from build123d import *

# Parameters (mm, degrees)
F0_W     = 27
F0_H     = 12.6
F1_DEPTH = 4
F3_DEPTH = 25
F4_R     = 2
F6_DEPTH = 2
F7_SIZE2 = 2
F7_SIZE  = 1.8


with BuildPart() as f1:
    # F0 (on Top) → F1 (new body)
    with BuildSketch(Plane.XY):
        with Locations((13.5, 6.3)):
            Rectangle(F0_W, F0_H)
    extrude(amount=F1_DEPTH)

    # F2 (on face) → F3 (cut)
    with BuildSketch(Plane.XY.offset(4)):
        Polygon((11.3033894163, 10), (0, 10), (0, 2.6), (11.3033894163, 2.6), (15, 6.1416643043), align=None)
    extrude(amount=-F3_DEPTH, mode=Mode.SUBTRACT)

    # F4
    f4_edges = [f1.edges().sort_by_distance(p)[0] for p in [
        (11.303389, 10, 2),
        (15, 6.141664, 2),
        (11.303389, 2.6, 2),
    ]]
    fillet(f4_edges, radius=F4_R)

    # F5 (on face) → F6 (cut)
    with BuildSketch(Plane.XY.offset(4)):
        with BuildLine():
            Line((27, 12.6), (13, 12.6))
            Line((13, 12.6), (19.9540073999, 7.1233526669))
            ThreePointArc((19.9540073999, 7.1233526669), (20.4114805586, 6.1676652225), (19.9334913588, 5.2220720186))
            Line((19.9334913588, 5.2220720186), (13, 0))
            Line((13, 0), (27, 0))
            Line((27, 0), (27, 12.6))
        make_face()
    extrude(amount=-F6_DEPTH, mode=Mode.SUBTRACT)

    # F7
    f7_edges = [f1.edges().sort_by_distance(p)[0] for p in [
        (27, 6.3, 0),
    ]]
    f7_side = f1.faces().sort_by_distance((27, 6.3, 1))[0]
    chamfer(f7_edges, length=F7_SIZE, length2=F7_SIZE2, reference=f7_side)


solid = f1.part
Read the model definition and answer for the solid it produces. Units are mm, in the model's axes. A direction names the side the tool comes from. Round coordinates to 2 decimals unless told otherwise and drop trailing zeros. Write each loop counter-clockwise with the first axis right and the second up, starting at its lowest first coordinate (ties: lowest second). Pieces come first, ordered by that corner, then holes. Notation, with made-up numbers: M 44,27.5 L 53,27.5 A13 ccw 53,49.5 Z; hole C 40,48 d2. An arc over 180 degrees is marked long. Use a Markdown table: item, result.
1) Straight lines are drawn through the part: line 1 along Y through (x, z) = (8, 0.7); line 2 along Z through (x, y) = (19, 8.75); line 3 along Y through (x, z) = (11.25, 2.7). For each, find the intervals that lie inside material, in ascending order. Write a range as [from, to].
Answers follow:
| item | result |
|---|---|
| line 1 | y = [0, 2.6], [10, 12.6] |
| line 2 | z = [0, 2] |
| line 3 | y = [0, 2.75], [9.83, 12.6] |
2) The part is cut by section B-B (z = 3.5). Write down the section's boundary in (x, y).
Answers follow:
| item | result |
|---|---|
| outline | M 0,0 L 13,0 L 19.93,5.22 A1.2 ccw 19.95,7.12 L 13,12.6 L 0,12.6 L 0,10 L 10.45,10 A2 cw 11.89,9.38 L 13.62,7.59 A2 cw 13.56,4.76 L 11.88,3.16 A2 cw 10.5,2.6 L 0,2.6 Z |
3) Flat-ended cylindrical pins translate along their axes: pin 1 (1.5 mm diameter, centred on y = 7, z = 0.5, fed in from -X); pin 2 (1.5 mm diameter, centred on x = 19, z = 3, fed in from +Y). Find the tip coordinate at first contact, or state that the pin passes through.
Answers follow:
| item | result |
|---|---|
| pin 1 | stops at x = 13.46 |
| pin 2 | stops at y = 8.47 |
4) The part is cut by section D-D (x = 16.5). Write down the section's boundary in (y, z).
Answers follow:
| item | result |
|---|---|
| outline | M 0,0 L 12.6,0 L 12.6,2 L 9.84,2 L 9.84,4 L 2.64,4 L 2.64,2 L 0,2 Z |
5) The part is cut by section A-A (x = 8.5). Write down the section's boundary in (y, z), plus the area to 3 significant figures.
Answers follow:
| item | result |
|---|---|
| outline | M 0,0 L 2.6,0 L 2.6,4 L 0,4 Z; M 10,0 L 12.6,0 L 12.6,4 L 10,4 Z |
| area | 20.8 mm2 |
6) For a pull along Y with two mould halves and no side action, classify faces 6 (the flat face through (16.52, 2.65, 3.01)), 7 (the flat face through (15, 6, 0)), 8 (the flat face through (12.71, 3.95, 2.03)) as pulls with the +Y half, pulls with the -Y half, needs draft (parallel to the pull), parting line crosses it, or undercut.
Answers follow:
| item | result |
|---|---|
| face 6 | pulls with the -Y half |
| face 7 | needs draft |
| face 8 | undercut |
7) A tool of negligible diameter and unlimited length cuts with its end or side. For faces 1 (the flat face through (16.43, 9.9, 3.01)), 2 (the cylindrical face through (20.41, 6.18, 3.01)), 3 (the flat face through (5, 2.6, 2)), 4 (the flat face through (26, 6.2, 0.9)), 5 (the flat face through (12.3, 9.2, 4)), from which of +Z, -Z, +X, -X, +Y, -Y can it reach the whole face along a straight path? Write none if from no direction.
Answers follow:
| item | result |
|---|---|
| face 1 | +Z, +X, +Y |
| face 2 | +Z, +X |
| face 3 | +Z, -Z, -X |
| face 4 | -Z, +X, +Y, -Y |
| face 5 | +Z, +X, -X, +Y, -Y |
8) The part is cut by section C-C (y = 4.25). Write down the section's boundary in (x, z).
Answers follow:
| item | result |
|---|---|
| outline | M 13.03,0 L 25,0 L 27,1.8 L 27,2 L 18.64,2 L 18.64,4 L 13.03,4 Z |
